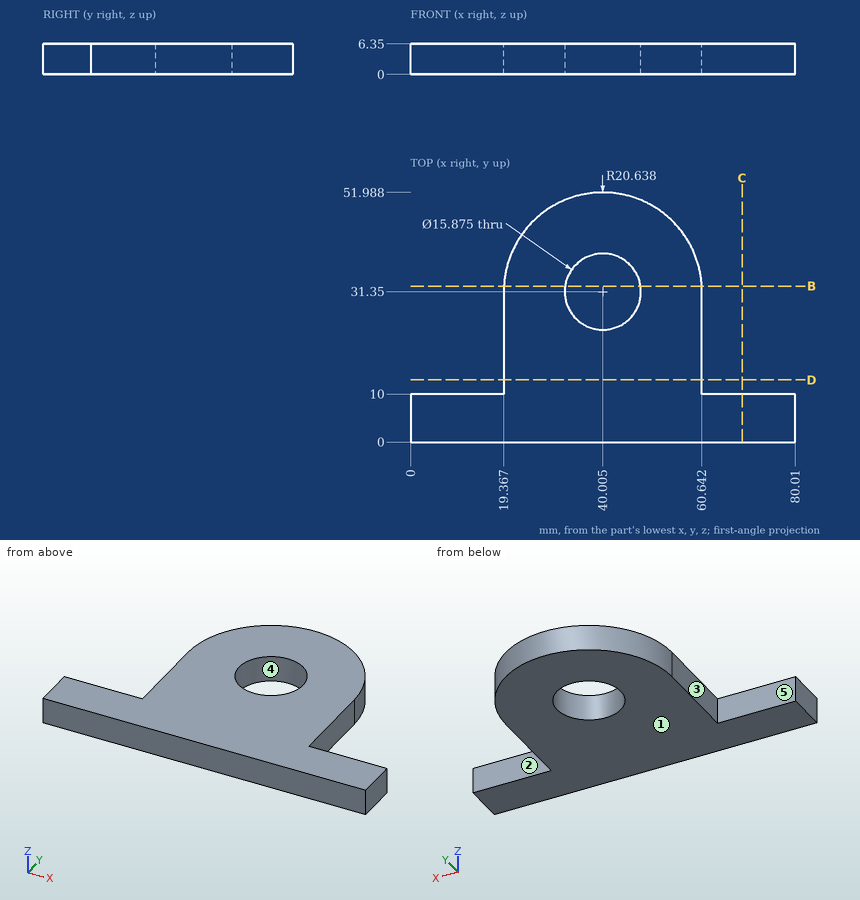
Input: dimensioned drawing with shaded views. Units: mm. Origin: part minimum x, y, z. A direction names the side the tool comes from. Give positions to 0.01 mm unless a question says otherwise; leave off trailing zeros. Write each loop counter-clockwise with the first axis right and the second up, starting at its lowest first coordinate (ties: lowest second). Pieces come first, ordered by that corner, then holes. Notation, with made-up numbers: (58, 22) - (67, 22) arc R7 ccw to (67, 33) - close; hole circle Ø3 at (58, -12.5). An arc over 180 degrees is marked (long way). Write item = value, one per line. Start each with the question number.
1) Draft query along X for the marked faces 3, 4 and 5. Return one class per face: pulls with the +X half, pulls with the -X half, needs draft (parallel to the pull), parting line crosses it, or undercut.
2) Cut plane B-B (y = 32.5). Return loops of the section in (x, z).
3) Cut plane C-C (x = 69). Return loops of the section in (y, z).
4) Cut plane D-D (y = 13). Return loops of the section in (x, z), and give its area (3 significant figures).
5) Reachability of the marked faces 1 and 2 from +Z, -Z, +X, -X, +Y, -Y: full face, straight path, thin tool, end or side. Return the list, or none.
6) Pin query (flat end, axial travel): pin 1 (3 mm diameter, centred on x = 10.5, z = 4.5, fed in from +Y). Return the tip coordinate at first contact, or that it passes through.
7) Material intervals for L1, parallel to X at y = 31.5, z = 2; L2, parallel to X at y = 18.5, z = 3; L3, parallel to Y at x = 69, z = 3.25, sorted ascending. Write a range as [from, to].
Answers follow:
q1.face_3 = pulls with the -X half
q1.face_4 = undercut
q1.face_5 = needs draft
q2.outline = (19.4, 0) - (32.15, 0) - (32.15, 6.35) - (19.4, 6.35) - close; (47.86, 0) - (60.61, 0) - (60.61, 6.35) - (47.86, 6.35) - close
q3.outline = (0, 0) - (10, 0) - (10, 6.35) - (0, 6.35) - close
q4.outline = (19.37, 0) - (60.64, 0) - (60.64, 6.35) - (19.37, 6.35) - close
q4.area = 262 mm^2
q5.face_1 = -Z, +X, -X, +Y, -Y
q5.face_2 = +Z, -Z, +X, +Y
q6.pin_1 = 10
q7.L1 = [19.37, 32.07], [47.94, 60.64]
q7.L2 = [19.37, 60.64]
q7.L3 = [0, 10]
